```python
from build123d import *

# Parameters (mm, degrees)
SKETCH1_W                    = 212
SKETCH1_H                    = 85
BASE_FLANGE1_DEPTH           = 2
CUT_EXTRUDE1_REACH           = 230.414
SKETCH6_W                    = 10
SKETCH6_H                    = 75
EDGE_FLANGE1_STRIP_W         = 9.4732
EDGE_FLANGE1_STRIP_H         = 2
EDGE_FLANGE1_STRIP_CUT_DEPTH = 192
EDGE_FLANGE1_DEPTH           = 192
EDGE_FLANGE2_STRIP_W         = 9.4732
EDGE_FLANGE2_STRIP_H         = 2
EDGE_FLANGE2_STRIP_CUT_DEPTH = 192
EDGE_FLANGE2_DEPTH           = 192
CUT_EXTRUDE2_START           = -2.7366
SKETCH13_R                   = 2.5
SKETCH13_W                   = 70
SKETCH13_H                   = 20
SKETCH13_W_2                 = 94
CUT_EXTRUDE2_DEPTH           = 2.7366
CUT_EXTRUDE3_START           = -2.7366
SKETCH14_W                   = 70
SKETCH14_H                   = 11.2634
CUT_EXTRUDE3_DEPTH           = 2.7366


# Sheet-metal steps are written as plain solids
with BuildPart() as part:
    # Sketch1 → Base-Flange1 (new body)
    with BuildSketch(Plane(origin=(0, 0, 0), x_dir=(1, 0, 0), z_dir=(0, 1, 0))):
        with Locations((106, 42.5)):
            Rectangle(SKETCH1_W, SKETCH1_H)
    extrude(amount=-BASE_FLANGE1_DEPTH)

    # Sketch6 → Cut-Extrude1 (cut, up to next)
    with BuildSketch(Plane(origin=(0, 0, 0), x_dir=(1, 0, 0), z_dir=(0, 1, 0)), mode=Mode.PRIVATE) as cut_extrude1_sk1:
        with Locations((5, 47.5)):
            Rectangle(SKETCH6_W, SKETCH6_H)
    cut_extrude1_tool1 = extrude(cut_extrude1_sk1.sketch, amount=-CUT_EXTRUDE1_REACH, mode=Mode.PRIVATE) & part.part
    # Sketch6 → Cut-Extrude1 (cut, up to next)
    with BuildSketch(Plane(origin=(0, 0, 0), x_dir=(1, 0, 0), z_dir=(0, 1, 0)), mode=Mode.PRIVATE) as cut_extrude1_sk2:
        with Locations((207, 47.5)):
            Rectangle(SKETCH6_W, SKETCH6_H)
    cut_extrude1_tool2 = extrude(cut_extrude1_sk2.sketch, amount=-CUT_EXTRUDE1_REACH, mode=Mode.PRIVATE) & part.part
    add(cut_extrude1_tool1.solids().sort_by_distance((5, 0, -47.5))[0], mode=Mode.SUBTRACT)
    add(cut_extrude1_tool2.solids().sort_by_distance((207, 0, -47.5))[0], mode=Mode.SUBTRACT)

    # Edge-Flange1 strip (across the edge) → Edge-Flange1 strip cut (cut)
    with BuildSketch(Plane(origin=(202, 0, -85), x_dir=(0, 0, 1), z_dir=(-1, 0, 0))):
        with Locations((-2, -1)):
            Rectangle(EDGE_FLANGE1_STRIP_W, EDGE_FLANGE1_STRIP_H)
    extrude(amount=EDGE_FLANGE1_STRIP_CUT_DEPTH, mode=Mode.SUBTRACT)

    # Edge-Flange1 section (across the edge) → Edge-Flange1 (add)
    with BuildSketch(Plane(origin=(202, 0, -85), x_dir=(0, 0, 1), z_dir=(-1, 0, 0))):
        with BuildLine():
            Line((0, 0.7366), (0, 10))
            Line((0, 10), (2, 10))
            Line((2, 10), (2, 0.7366))
            ThreePointArc((2, 0.7366), (2.215745145, 0.215745145), (2.7366, 0))
            Line((2.7366, 0), (2.7366, -2))
            ThreePointArc((2.7366, -2), (0.801531583, -1.198468417), (0, 0.7366))
        make_face()
    extrude(amount=EDGE_FLANGE1_DEPTH)

    # Edge-Flange2 strip (across the edge) → Edge-Flange2 strip cut (cut)
    with BuildSketch(Plane(origin=(202, 10, -83), x_dir=(0, -1, 0), z_dir=(-1, 0, 0))):
        with Locations((-4, -1)):
            Rectangle(EDGE_FLANGE2_STRIP_W, EDGE_FLANGE2_STRIP_H)
    extrude(amount=EDGE_FLANGE2_STRIP_CUT_DEPTH, mode=Mode.SUBTRACT)

    # Edge-Flange2 section (across the edge) → Edge-Flange2 (add)
    with BuildSketch(Plane(origin=(202, 10, -83), x_dir=(0, -1, 0), z_dir=(-1, 0, 0))):
        with BuildLine():
            Line((-2, 0.7366), (-2, 18))
            Line((-2, 18), (0, 18))
            Line((0, 18), (0, 0.7366))
            ThreePointArc((0, 0.7366), (0.215745145, 0.215745145), (0.7366, 0))
            Line((0.7366, 0), (0.7366, -2))
            ThreePointArc((0.7366, -2), (-1.198468417, -1.198468417), (-2, 0.7366))
        make_face()
    extrude(amount=EDGE_FLANGE2_DEPTH)

    # Sketch13 → Cut-Extrude2 (cut)
    with BuildSketch(Plane(origin=(0, 12, 0), x_dir=(1, 0, 0), z_dir=(0, 1, 0)).offset(CUT_EXTRUDE2_START)):
        with Locations(Location((125, 75.2634, 0), (0, 0, 270))):
            Circle(SKETCH13_R)
        with Locations(Location((17, 75.2634, 0), (0, 0, 270))):
            Circle(SKETCH13_R)
        with Locations((167, 75)):
            Rectangle(SKETCH13_W, SKETCH13_H)
        with Locations((71, 75)):
            Rectangle(SKETCH13_W_2, SKETCH13_H)
    extrude(amount=CUT_EXTRUDE2_DEPTH, mode=Mode.SUBTRACT)

    # Sketch14 → Cut-Extrude3 (cut)
    with BuildSketch(Plane(origin=(0, 0, -85), x_dir=(-1, 0, 0), z_dir=(0, 0, -1)).offset(CUT_EXTRUDE3_START)):
        with Locations((-167, 3.6317)):
            Rectangle(SKETCH14_W, SKETCH14_H)
    extrude(amount=CUT_EXTRUDE3_DEPTH, mode=Mode.SUBTRACT)


solid = part.part
```
Here's how the part is built. I have some questions about the finished solid (model axes, mm). A direction names the side the tool comes from. Give positions to 0.01 mm unless a question says otherwise; leave off trailing zeros. Order: outer loops, then holes, each group sorted by start corner. A loop starts at its lowest first (then second) coordinate and runs counter-clockwise, first axis right, second up. Notation, with made-up numbers: (65, 80) - (122, 80) arc R17 cw to (122, 88) - close; hole circle Ø9 at (-19, 72). An arc over 180 degrees is marked (long way). Answer as a JSON object with one key per item and string values. Group by question number.
Item 1: Please list where these lines run through material, in increasing order: probe 1 along Y at (x, z) = (23.5, -65.5); probe 2 along Y at (x, z) = (139, -77.5); probe 3 along Z at (x, y) = (96, 6.75).
Item 2: Which directions (+Z, -Z, +X, -X, +Y, -Y) give clear straight access to the entire face, cutting with the end or side of a thin tool? Please do faces 5 (the flat face through (72, 5, -85)), 6 (the cylindrical face through (127.48, 10.99, -75.59)), 7 (the flat face through (125, 10, -72)).
Item 3: If we mould it in two halves opening along X, with no side actions, what happens to faces 1 (the flat face through (10, -1, -56)), 2 (the flat face through (105, 0, -42)), 3 (the flat face through (132, 10.2, -77.9)), 4 (the cylindrical face through (18.69, 10.986, -77.106))? For each: pulls with the +X half, pulls with the -X half, needs draft (parallel to the pull), parting line crosses it, or undercut.
Item 4: If we section it at B-B on x = 103.5: Please give me the cut outline in (y, z).
Item 5: If we section it at A-A on x = 17: Please give me the cut outline in (y, z).
Item 6: If we section it at C-C on z = -27.5: Please give me the cut outline in (x, y), and give its area (3 significant figures).
Item 7: For P1, Ø1.6, axis at x = 19.5, y = 10.5, coming from the +Z side; P2, Ø3, axis at y = 10.5, z = -71, coming from the +X side; P3, Ø2, axis at y = 10, z = -70, coming from the -X side, each with a flat end and sliding along its axis, tell me the tip position at first contact or that it passes through.
Result set:
{
 "1": {"probe 1": "-2 to 0, 10 to 12", "probe 2": "-2 to 0", "probe 3": "-85 to -83"},
 "2": {"face 5": "-Z, +X, -X, +Y, -Y", "face 6": "+Y", "face 7": "+Z, +X, -X"},
 "3": {"face 1": "pulls with the -X half", "face 2": "needs draft", "face 3": "pulls with the +X half", "face 4": "undercut"},
 "4": {"outline": "(-2, -82.26) arc R2.74 ccw to (0.74, -85) - (9.26, -85) - (9.26, -83) - (0.74, -83) arc R0.74 cw to (0, -82.26) - (0, 0) - (-2, 0) - close"},
 "5": {"outline": "(-2, -82.26) arc R2.74 ccw to (0.74, -85) - (9.26, -85) arc R2.74 ccw to (12, -82.26) - (12, -77.76) - (10, -77.76) - (10, -82.26) arc R0.74 cw to (9.26, -83) - (0.74, -83) arc R0.74 cw to (0, -82.26) - (0, 0) - (-2, 0) - close; (10, -72.76) - (12, -72.76) - (12, -65) - (10, -65) - close"},
 "6": {"outline": "(10, -2) - (202, -2) - (202, 0) - (10, 0) - close", "area": "384 mm²"},
 "7": {"P1": "z = -65", "P2": "x = 132", "P3": "x = 10"}
}
